from build123d import *

# Parameters (mm, degrees)
F0_W     = 5
F0_H     = 80
F0_H_2   = 5
F0_W_2   = 70
F1_DEPTH = 60
F3_DEPTH = 85.001
F5_DEPTH = 80.001


with BuildPart() as f1:
    # F0 (on Front) → F1 (new body)
    with BuildSketch(Plane.XZ):
        with Locations((-37.5, -2.5)):
            Rectangle(F0_W, F0_H)
        with Locations((-37.5, 40)):
            Rectangle(F0_W, F0_H_2)
        with Locations((0, 40)):
            Rectangle(F0_W_2, F0_H_2)
        with Locations((37.5, 40)):
            Rectangle(F0_W, F0_H_2)
        with Locations((37.5, -2.5)):
            Rectangle(F0_W, F0_H)
    extrude(amount=F1_DEPTH)

    # F2 (on face) → F3 (cut, through all)
    with BuildSketch(Plane.XY.offset(42.5)):
        with BuildLine():
            Line((22.3145879042, -29.55), (23.0940107676, -30))
            Line((23.0940107676, -30), (22.3145879042, -30.45))
            ThreePointArc((22.3145879042, -30.45), (23.3269479082, -30.8693332437), (23.9940107676, -30))
            ThreePointArc((23.9940107676, -30), (23.3269479082, -29.1306667563), (22.3145879042, -29.55))
        make_face()
        with BuildLine():
            Line((22.3145879042, -30.45), (23.0940107676, -30))
            Line((23.0940107676, -30), (22.3145879042, -29.55))
            ThreePointArc((22.3145879042, -29.55), (22.1940107676, -30), (22.3145879042, -30.45))
        make_face()
        with BuildLine():
            ThreePointArc((-11.5470053838, -10.9), (-11.0970053838, -10.7794228634), (-10.7675825204, -10.45))
            Line((-10.7675825204, -10.45), (-11.5470053838, -10))
            Line((-11.5470053838, -10), (-11.5470053838, -10.9))
        make_face()
        with BuildLine():
            Line((-11.5470053838, -10), (-10.7675825204, -10.45))
            ThreePointArc((-10.7675825204, -10.45), (-10.6776721401, -10.2329371406), (-10.6470053838, -10))
            ThreePointArc((-10.6470053838, -10), (-12.1834014869, -9.3636038969), (-11.5470053838, -10.9))
            Line((-11.5470053838, -10.9), (-11.5470053838, -10))
        make_face()
        with BuildLine():
            Line((-11.5470053838, -50), (-10.7675825204, -49.55))
            ThreePointArc((-10.7675825204, -49.55), (-11.0970053838, -49.2205771366), (-11.5470053838, -49.1))
            Line((-11.5470053838, -49.1), (-11.5470053838, -50))
        make_face()
        with BuildLine():
            ThreePointArc((-10.6470053838, -50), (-10.6776721401, -49.7670628594), (-10.7675825204, -49.55))
            Line((-10.7675825204, -49.55), (-11.5470053838, -50))
            Line((-11.5470053838, -50), (-11.5470053838, -49.1))
            ThreePointArc((-11.5470053838, -49.1), (-12.1834014869, -50.6363961031), (-10.6470053838, -50))
        make_face()
    extrude(amount=-F3_DEPTH, mode=Mode.SUBTRACT)

    # F4 (on face) → F5 (cut, through all)
    with BuildSketch(Plane.YZ.offset(40)):
        Polygon((-60, -42.5), (-30, -42.5), (-60, 42.5), align=None)
        Polygon((0, 42.5), (-30, -42.5), (0, -42.5), align=None)
    extrude(amount=-F5_DEPTH, mode=Mode.SUBTRACT)


solid = f1.part
Here's how the part is built. I have some questions about the finished solid (model axes, mm). A direction names the side the tool comes from. Give positions to 0.01 mm unless a question says otherwise; leave off trailing zeros. Loops run counter-clockwise (first coordinate to the right, second up) from the corner with the lowest first, then second, coordinate; pieces in that order, holes last. Notation, with made-up numbers: (39, 38.25) -> (49, 38.25) arc R32 ccw to (49, 76.25) -> close; hole circle Ø7 at (30, -16.75). An arc over 180 degrees is marked (long way). Answer as a JSON object with one key per item and string values. Group by question number.
Item 1: Will these pins go through, and if not, where does the flat tip stop? pin 1 (17 mm diameter, centred on x = -1.5, y = -22, fed in from -Z); pin 2 (1.4 mm diameter, centred on x = -11.55, y = -10, fed in from +Z).
Item 2: Imagine slicing it at B-B on y = -27. Write out the boundary of the cut face in (x, z).
Item 3: Thinking about a two-plate mould opening in X: for faces 3 (the flat face through (-2.776, -1.597, 37.976)), 4 (the flat face through (-35, -30, 6)), 5 (the flat face through (40, -30, 9)), which applies, pulls with the +X half, pulls with the -X half, needs draft (parallel to the pull), parting line crosses it, or undercut?
Item 4: Imagine slicing it at A-A on z = 17. Write out the boundary of the cut face in (x, y).
Item 5: Imagine slicing it at D-D on z = -36.5. Write out the boundary of the cut face in (x, y), then the cut area to 3 significant figures.
Item 6: On a 3-axis mill with a long thin cutter (end or side, diameter ignored), from which of +Z, -Z, +X, -X, +Y, -Y can I reach the whole of each face in a straight line? I mean faces 1 (the flat face through (1, -30, 42.5)), 2 (the flat face through (35, -30, 6)). Say none if no direction works.
Item 7: I need wall thicknesses on L1, parallel to X at y = -10, z = 41; L2, parallel to X at y = -33.5, z = -5; L3, parallel to Z at x = 20, y = -7. Which ranges of each line are inside material? Lowest first, please.
Item 8: Imagine slicing it at C-C on x = -14. Write out the boundary of the cut face in (y, z).
Answer list:
{
 "1": {"pin 1": "stops at z = 37.5", "pin 2": "passes through"},
 "2": {"outline": "(-40, -34) -> (-35, -34) -> (-35, 37.5) -> (35, 37.5) -> (35, -34) -> (40, -34) -> (40, 42.5) -> (-40, 42.5) -> close"},
 "3": {"face 3": "needs draft", "face 4": "undercut", "face 5": "pulls with the +X half"},
 "4": {"outline": "(-40, -51) -> (-35, -51) -> (-35, -9) -> (-40, -9) -> close; (35, -51) -> (40, -51) -> (40, -9) -> (35, -9) -> close"},
 "5": {"outline": "(-40, -32.12) -> (-35, -32.12) -> (-35, -27.88) -> (-40, -27.88) -> close; (35, -32.12) -> (40, -32.12) -> (40, -27.88) -> (35, -27.88) -> close", "area": "42.4 mm2"},
 "6": {"face 1": "+Z, +X, -X, +Y, -Y", "face 2": "-Z, +Y, -Y"},
 "7": {"L1": "x = -40 to -12.45, -10.65 to 40", "L2": "x = -40 to -35, 35 to 40", "L3": "z = 37.5 to 42.5"},
 "8": {"outline": "(-60, 42.5) -> (-58.24, 37.5) -> (-1.76, 37.5) -> (0, 42.5) -> close"}
}
